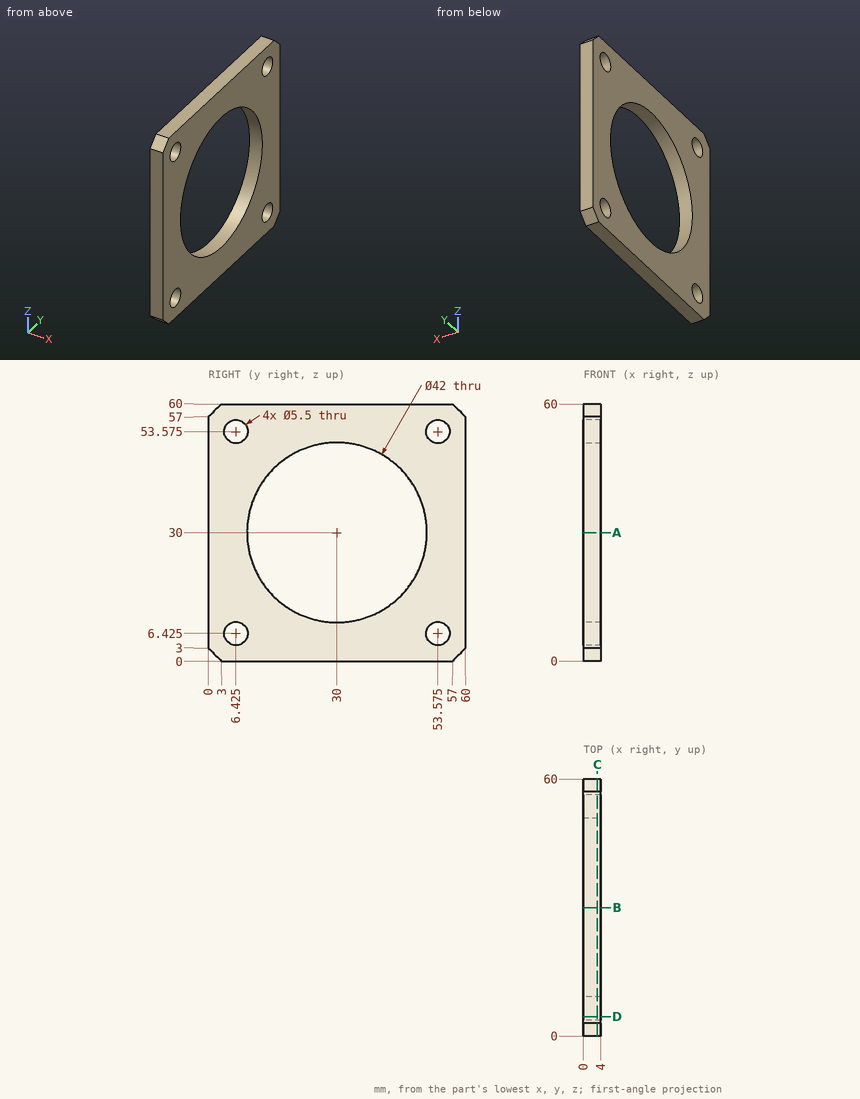
Can you work these out from the drawing? Everything is in mm from the part's minimum corner. Give positions to 0.01 mm unless a question says otherwise; leave off trailing zeros. Loops run counter-clockwise (first coordinate to the right, second up) from the corner with the lowest first, then second, coordinate; pieces in that order, holes last. Notation, with made-up numbers: (56, 73.5) - (83, 73.5) arc R13 cw to (83, 84.5) - close; hole circle Ø10 at (48.25, 17). An arc over 180 degrees is marked (long way). Use one line per item in the form item = value.
1. I'm going to push a flat-ended pin straight in: pin 1 Ø6.5 at (y, z) = (53.575, 53.575) entering from +X. Where does the tip first touch, or does it pass through?
Response values:
pin_1 = 4
2. I need wall thicknesses on probe 1 along Z at (x, y) = (1.9, 4); probe 2 along Y at (x, z) = (1.15, 30); probe 3 along Y at (x, z) = (0.5, 48). Which ranges of each line are inside material? Lowest first, please.
Response values:
probe_1 = 0 to 5.13, 7.72 to 52.28, 54.87 to 60
probe_2 = 0 to 9, 51 to 60
probe_3 = 0 to 19.18, 40.82 to 60
3. I want a section at A-A (z = 30). Please give me the cut outline in (x, y), and give its area (3 significant figures).
Response values:
outline = (0, 0) - (4, 0) - (4, 9) - (0, 9) - close; (0, 51) - (4, 51) - (4, 60) - (0, 60) - close
area = 72.0 mm²
4. I want a section at D-D (y = 4.5). Please give me the cut outline in (x, z).
Response values:
outline = (0, 0) - (4, 0) - (4, 4.46) - (0, 4.46) - close; (0, 8.39) - (4, 8.39) - (4, 51.61) - (0, 51.61) - close; (0, 55.54) - (4, 55.54) - (4, 60) - (0, 60) - close
5. I want a section at C-C (x = 3.25). Please give me the cut outline in (y, z) (3 decimals).
Response values:
outline = (0, 3) - (3, 0) - (57, 0) - (60, 3) - (60, 57) - (57, 60) - (3, 60) - (0, 57) - close; hole circle Ø5.5 at (6.425, 6.425); hole circle Ø5.5 at (6.425, 53.575); hole circle Ø42 at (30, 30); hole circle Ø5.5 at (53.575, 6.425); hole circle Ø5.5 at (53.575, 53.575)
